```python
from build123d import *

# Parameters (mm, degrees)
F2_DEPTH = 14.5
F0_R     = 1.65
F3_DEPTH = 15


# Not quite as in the source:
# - the program builds the solid bodies; features that only make, move or delete a surface that nothing else refers to are left out


with BuildPart() as f2:
    # F0 (on Top) → F2 (new body, symmetric)
    with BuildSketch(Plane.XY):
        with BuildLine():
            ThreePointArc((-2.4681723606, -1.4250000696), (-2.85, -3.73e-08), (-2.4681723979, 1.425000005))
            Line((-2.4681723979, 1.425000005), (-3.2908965344, 0))
            Line((-3.2908965344, 0), (-2.4681723606, -1.4250000696))
        make_face()
    extrude(amount=F2_DEPTH, both=True)



with BuildPart() as f2b:
    # F0 (on Top) → F2, piece 2 (new body, symmetric)
    with BuildSketch(Plane.XY):
        with BuildLine():
            ThreePointArc((-2.4681723979, 1.425000005), (-1.4249999975, 2.4681724022), (0, 2.85))
            Line((0, 2.85), (-1.6454482672, 2.85))
            Line((-1.6454482672, 2.85), (-2.4681723979, 1.425000005))
        make_face()
    extrude(amount=F2_DEPTH, both=True)


with BuildPart() as f2c:
    # F0 (on Top) → F2, piece 3 (new body, symmetric)
    with BuildSketch(Plane.XY):
        with BuildLine():
            ThreePointArc((0, 2.85), (1.4249999814, 2.4681724115), (2.4681723793, 1.4250000373))
            Line((2.4681723793, 1.4250000373), (1.6454482672, 2.85))
            Line((1.6454482672, 2.85), (0, 2.85))
        make_face()
    extrude(amount=F2_DEPTH, both=True)


with BuildPart() as f2d:
    # F0 (on Top) → F2, piece 4 (new body, symmetric)
    with BuildSketch(Plane.XY):
        with BuildLine():
            ThreePointArc((2.4681723793, 1.4250000373), (2.7528885994, 0.7376342993), (2.85, 0))
            ThreePointArc((2.85, 0), (2.7528886042, -0.7376342813), (2.4681723979, -1.425000005))
            Line((2.4681723979, -1.425000005), (3.2908965344, 0))
            Line((3.2908965344, 0), (2.4681723793, 1.4250000373))
        make_face()
    extrude(amount=F2_DEPTH, both=True)


with BuildPart() as f2e:
    # F0 (on Top) → F2, piece 5 (new body, symmetric)
    with BuildSketch(Plane.XY):
        with BuildLine():
            Line((1.6454482672, -2.85), (2.4681723979, -1.425000005))
            ThreePointArc((2.4681723979, -1.425000005), (1.4249999975, -2.4681724022), (0, -2.85))
            Line((0, -2.85), (1.6454482672, -2.85))
        make_face()
    extrude(amount=F2_DEPTH, both=True)


with BuildPart() as f2f:
    # F0 (on Top) → F2, piece 6 (new body, symmetric)
    with BuildSketch(Plane.XY):
        with BuildLine():
            Line((-1.6454482672, -2.85), (0, -2.85))
            ThreePointArc((0, -2.85), (-1.4249999652, -2.4681724209), (-2.4681723606, -1.4250000696))
            Line((-2.4681723606, -1.4250000696), (-1.6454482672, -2.85))
        make_face()
    extrude(amount=F2_DEPTH, both=True)


with BuildPart() as f2_1:
    add(f2.part)

    add(f2b.part)  # F3 merges F2b

    add(f2c.part)  # F3 merges F2c

    add(f2d.part)  # F3 merges F2d

    add(f2e.part)  # F3 merges F2e

    add(f2f.part)  # F3 merges F2f
    # F0 (on Top) → F3 (join, symmetric)
    with BuildSketch(Plane.XY):
        with BuildLine():
            ThreePointArc((2.4681723979, -1.425000005), (2.7528886042, -0.7376342813), (2.85, 0))
            ThreePointArc((2.85, 0), (2.7528885994, 0.7376342993), (2.4681723793, 1.4250000373))
            ThreePointArc((2.4681723793, 1.4250000373), (1.4249999814, 2.4681724115), (0, 2.85))
            ThreePointArc((0, 2.85), (-1.4249999975, 2.4681724022), (-2.4681723979, 1.425000005))
            ThreePointArc((-2.4681723979, 1.425000005), (-2.85, -3.73e-08), (-2.4681723606, -1.4250000696))
            ThreePointArc((-2.4681723606, -1.4250000696), (-1.4249999652, -2.4681724209), (0, -2.85))
            ThreePointArc((0, -2.85), (1.4249999975, -2.4681724022), (2.4681723979, -1.425000005))
        make_face()
        Circle(F0_R, mode=Mode.SUBTRACT)
    extrude(amount=F3_DEPTH, both=True)


solid = f2_1.part
```
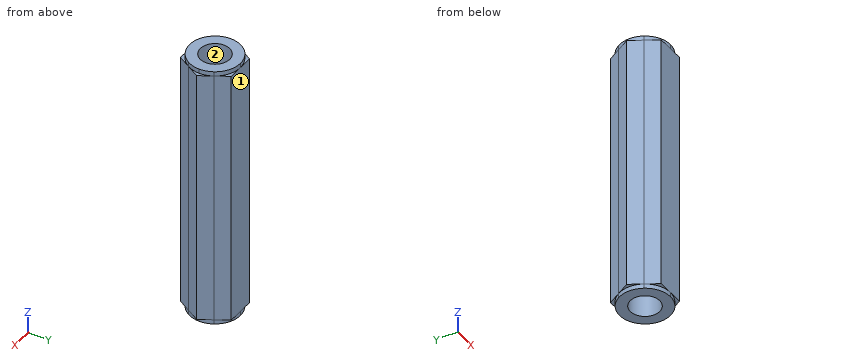
Design review of the part built by this model. Coordinates are the model's own, in mm. Face numbers are marked on the shaded views. Coordinates: 2 decimals unless noted, no trailing zeros. Order: outer loops, then holes, each group sorted by start corner. A loop starts at its lowest first (then second) coordinate and runs counter-clockwise, first axis right, second up. Notation, with made-up numbers: M -26.5,51 L 1.5,51 A17 ccw 1.5,83 Z; hole C 4,11.25 d6. An arc over 180 degrees is marked long. Answer as a JSON object with one key per item and string values. Group by question number.
1) Add section C-C, the plane x = 0.5. Write out the cut boundary in (y, z).
2) For pin 1 (0.7 mm diameter, centred on x = 3, y = 0.5, fed in from -Z); pin 2 (3 mm diameter, centred on x = 0, y = 0, fed in from -Z); pin 3 (2 mm diameter, centred on y = 1.5, z = -11, fed in from -X); pin 4 (1.5 mm diameter, centred on y = -1.5, z = -0.5, fed in from +X), all flat-tipped, find the tip position at first contact; note any pin that passes through.
3) Wall thickness on L1, parallel to X at y = -0.9, z = 11; L2, parallel to Y at x = -0.5, z = 9; L3, parallel to Z at x = -1.75, y = 2.45: over which ranges is each line inside the solid? List them lowest first.
4) Mouldability with a two-part tool opening along X and no side actions: class the marked faces 1 and 2 as pulls with the +X half, pulls with the -X half, needs draft (parallel to the pull), parting line crosses it, or undercut.
5) Add section A-A, the plane y = -0.75. Write out the cut boundary in (x, z).
6) Add section B-B, the plane z = 7.5. Write out the cut boundary in (x, y) (3 decimals).
7) Add section D-D, the plane y = -2.05. Write out the cut boundary in (x, z), then the cut area to 3 significant figures.
Computed values:
{
 "1": {"outline": "M -2.85,-14.5 L -2.81,-14.5 L -2.81,-15 L -1.57,-15 L -1.57,15 L -2.81,15 L -2.81,14.5 L -2.85,14.5 Z; M 1.57,-15 L 2.81,-15 L 2.81,-14.5 L 2.85,-14.5 L 2.85,14.5 L 2.81,14.5 L 2.81,15 L 1.57,15 Z"},
 "2": {"pin 1": "stops at z = -15", "pin 2": "passes through", "pin 3": "stops at x = -3", "pin 4": "stops at x = 2.86"},
 "3": {"L1": "x = -2.77 to -1.38, 1.38 to 2.77", "L2": "y = -2.85 to -1.57, 1.57 to 2.85", "L3": "z = -14.5 to 14.5"},
 "4": {"face 1": "needs draft", "face 2": "undercut"},
 "5": {"outline": "M -2.86,-14.5 L -2.75,-14.5 L -2.75,-15 L -1.47,-15 L -1.47,15 L -2.75,15 L -2.75,14.5 L -2.86,14.5 Z; M 1.47,-15 L 2.75,-15 L 2.75,-14.5 L 2.86,-14.5 L 2.86,14.5 L 2.75,14.5 L 2.75,15 L 1.47,15 Z"},
 "6": {"outline": "M -3.291,0 L -1.645,-2.85 L 1.645,-2.85 L 3.291,0 L 1.645,2.85 L -1.645,2.85 Z; hole C 0,0 d3.3"},
 "7": {"outline": "M -2.11,-14.5 L -1.98,-14.5 L -1.98,-15 L 1.98,-15 L 1.98,-14.5 L 2.11,-14.5 L 2.11,14.5 L 1.98,14.5 L 1.98,15 L -1.98,15 L -1.98,14.5 L -2.11,14.5 Z", "area": "126 mm^2"}
}
